Verification items for this drawing (mm, ordinates from the low corner). A direction names the side the tool comes from. Give positions to 0.01 mm unless a question says otherwise; leave off trailing zeros. Loops run counter-clockwise (first coordinate to the right, second up) from the corner with the lowest first, then second, coordinate; pieces in that order, holes last. Notation, with made-up numbers: M -11,-17.75 L 34,-17.75 A13 cw 34,-9.75 Z; hole C 61.5,29 d5. An arc over 180 degrees is marked long. Use one line per item in the form item = value.
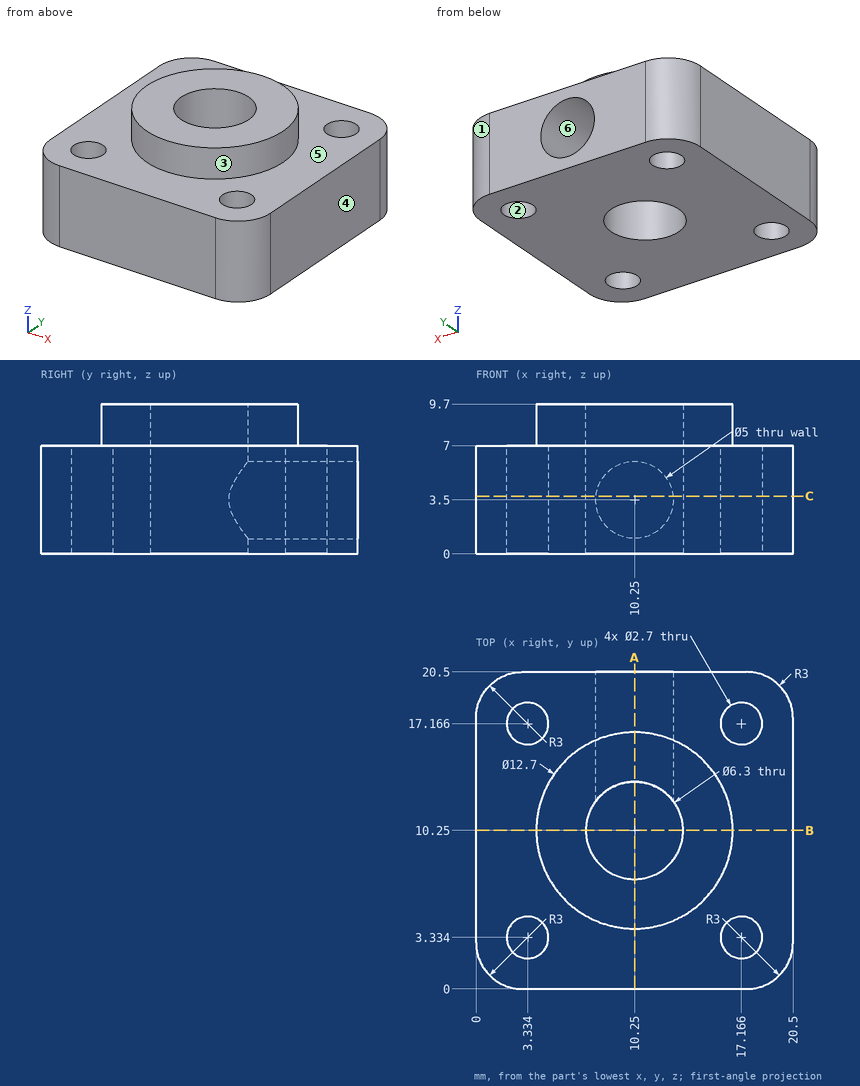
1) Section check A-A (x = 10.25). Record the cut outline in (y, z).
Evaluation:
outline = M 0,0 L 7.1,0 L 7.1,9.7 L 3.9,9.7 L 3.9,7 L 0,7 Z; M 13.4,0 L 20.5,0 L 20.5,1 L 13.4,1 Z; M 13.4,6 L 20.5,6 L 20.5,7 L 16.6,7 L 16.6,9.7 L 13.4,9.7 Z
2) Section check B-B (y = 10.25). Record the cut outline in (x, z), then the cut area to 3 significant figures.
Evaluation:
outline = M 0,0 L 7.1,0 L 7.1,9.7 L 3.9,9.7 L 3.9,7 L 0,7 Z; M 13.4,0 L 20.5,0 L 20.5,7 L 16.6,7 L 16.6,9.7 L 13.4,9.7 Z
area = 117 mm^2
3) Scan lines: line 1 (X direction, y = 2.25, z = 4.25) (1 decimal); line 2 (X direction, y = 4.25, z = 1.75) (1 decimal); line 3 (Y direction, x = 2.75, z = 2.5). Record each from-to range of solid material in increasing order.
Evaluation:
line_1 = 0.1 to 2.5, 4.1 to 16.4, 18 to 20.4
line_2 = 0 to 2.3, 4.3 to 16.2, 18.2 to 20.5
line_3 = 0.01 to 2.12, 4.55 to 15.95, 18.38 to 20.49
4) Depth check by flat-ended pin: pin 1 Ø1.6 at (x, y) = (17.17, 3.33) entering from -Z; pin 2 Ø4 at (x, y) = (2.5, 6.5) entering from +Z. Enter the tip coordinate at first touch or a pass-through.
Evaluation:
pin_1 = through
pin_2 = 7
5) Section check C-C (z = 3.75). State how many separate pieces and enclosed holes the cut face has, then the cut area to 3 significant figures.
Evaluation:
separate_pieces = 1
enclosed_holes = 4
area = 321 mm^2
6) Release check for a two-part mould opening along Y. For the marked faces 1, 2 and 3 record: pulls with the +Y half, pulls with the -Y half, needs draft (parallel to the pull), parting line crosses it, or undercut.
Evaluation:
face_1 = pulls with the +Y half
face_2 = undercut
face_3 = parting line crosses it
7) Set-up check for the marked faces 4, 5 and 6: record each of +Z, -Z, +X, -X, +Y, -Y from which the full face is reachable in a straight line by a thin tool's end or side.
Evaluation:
face_4 = +Z, -Z, +X, +Y, -Y
face_5 = +Z
face_6 = +Y
